Input: dimensioned drawing with shaded views. Units: mm. Origin: part minimum x, y, z. Give positions to 0.01 mm unless a question says otherwise; leave off trailing zeros. Order: outer loops, then holes, each group sorted by start corner. A loop starts at its lowest first (then second) coordinate and runs counter-clockwise, first axis right, second up. Notation, with made-up numbers: (-10.5, 61) -> (2.5, 61) arc R24 ccw to (2.5, 86) -> close; hole circle Ø6 at (61, -13.5). An arc over 180 degrees is marked (long way). Use CSV: the item, a comma, the result in double quotes.
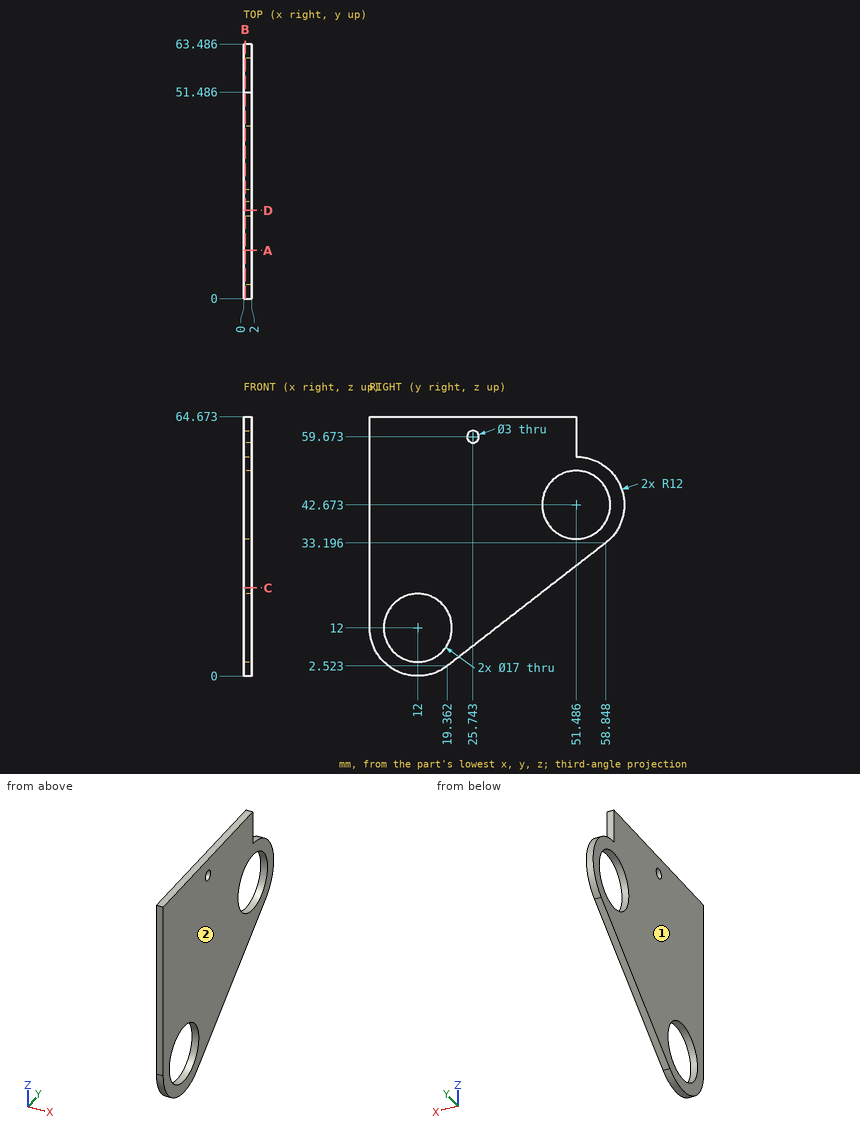
1. Mould query, pull axis X, two halves, no side actions, for the marked faces 1 and 2. Classes: released by +X, released by -X, zero draft, split by the parting line, or undercut.
Answer below:
face 1,"released by -X"
face 2,"released by +X"
2. Section query A-A on y = 12. Return loops of the section in (x, z).
Answer below:
outline,"(0, 0) -> (2, 0) -> (2, 3.5) -> (0, 3.5) -> close; (0, 20.5) -> (2, 20.5) -> (2, 64.67) -> (0, 64.67) -> close"
3. Section query B-B on x = 0.35. Return loops of the section in (y, z).
Answer below:
outline,"(0, 12) arc R12 ccw to (19.36, 2.52) -> (58.85, 33.2) arc R12 ccw to (51.49, 54.67) -> (51.49, 64.67) -> (0, 64.67) -> close; hole circle Ø17 at (12, 12); hole circle Ø3 at (25.74, 59.67); hole circle Ø17 at (51.49, 42.67)"
4. Section query D-D on y = 22. Return loops of the section in (x, z).
Answer below:
outline,"(0, 4.57) -> (2, 4.57) -> (2, 64.67) -> (0, 64.67) -> close"
5. Ray query, line 1 along Z through (x, y) = (1.65, 8) (1 decimal); line 2 along Y through (x, z) = (1.6, 7) (1 decimal); line 3 along Y through (x, z) = (0.1, 37) (1 decimal). Return the intervals inside material, ascending.
Answer below:
line 1,"z = 0.7 to 4.5, 19.5 to 64.7"
line 2,"y = 1.1 to 5.1, 18.9 to 25.1"
line 3,"y = 0 to 45.2, 57.8 to 62.1"
6. Section query C-C on z = 22. Return loops of the section in (x, y) (1 decimal).
Answer below:
outline,"(0, 0) -> (2, 0) -> (2, 44.4) -> (0, 44.4) -> close"
